Geometry: final body of the model. Coordinates: model frame, mm. Coordinates: 2 decimals unless noted, no trailing zeros. Loops run counter-clockwise (first coordinate to the right, second up) from the corner with the lowest first, then second, coordinate; pieces in that order, holes last. Notation, with made-up numbers: (55.5, 10) -> (61.5, 10) arc R28 ccw to (61.5, 47) -> close; hole circle Ø10 at (-8.75, 88.25). An arc over 180 degrees is marked (long way). One line per item, written item: value. Start each with the question number.
Item 1: Section query A-A on z = 22.5. Return loops of the section in (x, y).
Item 2: Section query B-B on y = -9.5. Return loops of the section in (x, z) (3 decimals), then the cut area to 4 significant figures.
Item 3: Section query D-D on z = -16. Return loops of the section in (x, y).
Item 4: Section query C-C on x = 0.7. Give the number of separate pieces and of enclosed holes in the cut face, then the cut area to 3 significant figures.
Item 5: Contact query for flat-ended pins moving along their axis: pin 1 Ø0.8 at (x, z) = (1, 17) entering from -Y; pin 2 Ø1 at (x, z) = (2, -32) entering from +Y. Output: stop coordinate, or through.
Item 6: Ray query, probe 1 along Z at (x, y) = (2.25, 13) (3 decimals); probe 2 along Y at (x, z) = (2.25, 29.5). Return the intervals inside material, ascending. Write a range as from..to.
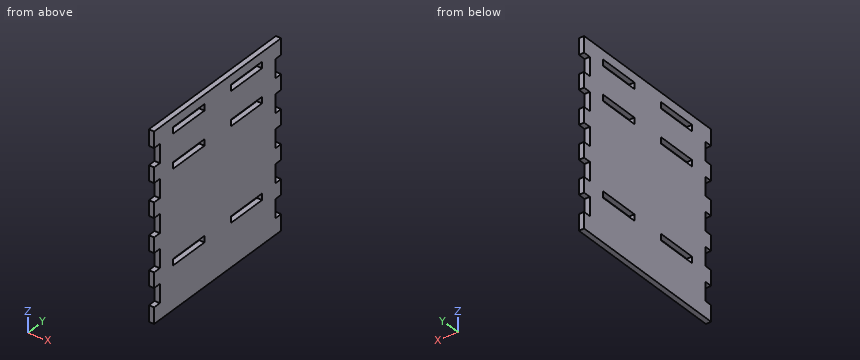
from build123d import *

# Parameters (mm, degrees)
F0_W     = 3.6
F0_H     = 7.6
F0_H_2   = 7.2
F0_W_2   = 19.7
F0_H_3   = 3
F1_DEPTH = 2.5


# Not quite as in the source:
# - a feature names something its author has since deleted; it is built from what else it names


with BuildPart() as f1:
    # F0 (on Right) → F1 (new body)
    with BuildSketch(Plane.YZ):
        with Locations((38.2, -40.2)):
            Rectangle(F0_W, F0_H)
        with Locations((-38.2, -40.2)):
            Rectangle(F0_W, F0_H)
        with Locations((38.2, 40.2)):
            Rectangle(F0_W, F0_H)
        with Locations((-38.2, 40.2)):
            Rectangle(F0_W, F0_H)
        with Locations((38.2, -8)):
            Rectangle(F0_W, F0_H_2)
        with Locations((-38.2, -8)):
            Rectangle(F0_W, F0_H_2)
        Polygon((-36.4, -36.4), (-36.4, -44), (36.4, -44), (36.4, -36.4), (36.4, -27.6), (36.4, -20.4), (36.4, -11.6), (36.4, -4.4), (36.4, 4.4), (36.4, 11.6), (36.4, 20.4), (36.4, 27.6), (36.4, 36.4), (36.4, 44), (-36.4, 44), (-36.4, 36.4), (-36.4, 27.6), (-36.4, 20.4), (-36.4, 11.6), (-36.4, 4.4), (-36.4, -4.4), (-36.4, -11.6), (-36.4, -20.4), (-36.4, -27.6), align=None)
        with Locations((-18.148, -22.104)):
            Rectangle(F0_W_2, F0_H_3, mode=Mode.SUBTRACT)
        with Locations((18.148, -22.104)):
            Rectangle(F0_W_2, F0_H_3, mode=Mode.SUBTRACT)
        with Locations((-18.148, 22.095)):
            Rectangle(F0_W_2, F0_H_3, mode=Mode.SUBTRACT)
        with Locations((-18.148, 38.1555415094)):
            Rectangle(F0_W_2, F0_H_3, mode=Mode.SUBTRACT)
        with Locations((18.148, 22.095)):
            Rectangle(F0_W_2, F0_H_3, mode=Mode.SUBTRACT)
        with Locations((18.148, 38.1555415094)):
            Rectangle(F0_W_2, F0_H_3, mode=Mode.SUBTRACT)
        with Locations((38.2, -24)):
            Rectangle(F0_W, F0_H_2)
        with Locations((-38.2, -24)):
            Rectangle(F0_W, F0_H_2)
        with Locations((38.2, 8)):
            Rectangle(F0_W, F0_H_2)
        with Locations((-38.2, 24)):
            Rectangle(F0_W, F0_H_2)
        with Locations((38.2, 24)):
            Rectangle(F0_W, F0_H_2)
        with Locations((-38.2, 8)):
            Rectangle(F0_W, F0_H_2)
    extrude(amount=F1_DEPTH)


solid = f1.part
Reply:
1. outline: (0, -40) -> (2.5, -40) -> (2.5, -28) -> (0, -28) -> close; (0, -8.3) -> (2.5, -8.3) -> (2.5, 8.3) -> (0, 8.3) -> close; (0, 28) -> (2.5, 28) -> (2.5, 40) -> (0, 40) -> close
2. outline: (0, -44) -> (2.5, -44) -> (2.5, -23.604) -> (0, -23.604) -> close; (0, -20.604) -> (2.5, -20.604) -> (2.5, 20.595) -> (0, 20.595) -> close; (0, 23.595) -> (2.5, 23.595) -> (2.5, 36.656) -> (0, 36.656) -> close; (0, 39.656) -> (2.5, 39.656) -> (2.5, 44) -> (0, 44) -> close
2. area: 197.5 mm²
3. outline: (0, -36.4) -> (2.5, -36.4) -> (2.5, 36.4) -> (0, 36.4) -> close
4. separate pieces: 1
4. enclosed holes: 6
4. area: 6,370 mm²
5. pin 1: stops at y = -36.4
5. pin 2: stops at y = 36.4
6. probe 1: z = -44..-23.604, -20.604..20.595, 23.595..36.656, 39.656..44
6. probe 2: y = -36.4..36.4
